from build123d import *

# Parameters (mm, degrees)
F1_DEPTH = 2.54
F2_R     = 1.27
F3_DEPTH = 25.4
F4_DEPTH = 6.35


with BuildPart() as f1:
    # F0 (on Top) → F1 (new body)
    with BuildSketch(Plane.XY):
        with BuildLine():
            Line((-17.6407694817, 88.9), (-3.0585505724, 88.9))
            ThreePointArc((-3.0585505724, 88.9), (-10.349660027, 95.0651364676), (-17.6407694817, 88.9))
        make_face()
        Polygon((-10.349660027, 0), (2.350339973, 0), (2.350339973, 56.8060912192), (-3.0585505724, 88.9), (-17.6407694817, 88.9), (-23.049660027, 56.8060912192), (-23.049660027, 0), align=None)
    extrude(amount=F1_DEPTH)

    # F2 (on face) → F3 (cut)
    with BuildSketch(Plane.XY.offset(2.54)):
        with Locations((-16.699660027, 6.35)):
            Circle(F2_R)
        with BuildLine():
            ThreePointArc((-2.729660027, 6.35), (-3.999660027, 7.62), (-5.269660027, 6.35))
            ThreePointArc((-5.269660027, 6.35), (-3.999660027, 5.08), (-2.729660027, 6.35))
        make_face()
    extrude(amount=-F3_DEPTH, mode=Mode.SUBTRACT)

    # F4 (add): a face of the model
    f4_faces = [f1.faces().sort_by_distance(p)[0] for p in [
        (-10.349660027, 0, 1.27),
    ]]
    extrude(f4_faces, amount=F4_DEPTH)


solid = f1.part
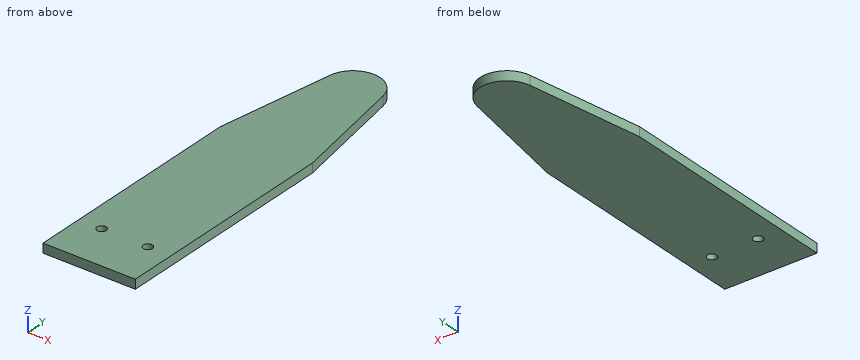
CAD build for the part. Positions are in the model's coordinates, mm. Coordinates: 2 decimals unless noted, no trailing zeros. Write each loop counter-clockwise with the first axis right and the second up, starting at its lowest first coordinate (ties: lowest second). Pieces come first, ordered by that corner, then holes. Notation, with made-up numbers: (0.5, -15) - (57.5, -15) arc R27 cw to (57.5, 1) - close; hole circle Ø1 at (59.25, 54.5). An arc over 180 degrees is marked (long way). Use a Markdown table: item, result. Add a question column.
Item 1: Flat gauge pin, fed straight in: pin 1 (1.5 mm diameter, centred on x = -16.7, y = 6.35, fed in from -Z). Where does the tip first touch, or does it go through?
Item 2: Band-saw the part on C-C, the plane x = -20.25. Give the cut face in (y, z).
Item 3: Band-saw the part on A-A, the plane y = 6.35. Give the cut face in (x, z).
Item 4: Drill centre lines: L1, parallel to Y at x = -4, z = 0.5; L2, parallel to Y at x = -17, z = 2.1; L3, parallel to Y at x = -8, z = 2.1. Where is each one in solid material? Low to high. Write a range as from..to.
Item 5: Band-saw the part on B-B, the plane z = 0.55. Give the cut face in (x, y), and give its area (3 significant figures).
Numbers:
| question | item | result |
|---|---|---|
| 1 | pin 1 | through |
| 2 | outline | (-6.35, 0) - (73.42, 0) - (73.42, 2.54) - (-6.35, 2.54) - close |
| 3 | outline | (-23.05, 0) - (-17.97, 0) - (-17.97, 2.54) - (-23.05, 2.54) - close; (-15.43, 0) - (-5.27, 0) - (-5.27, 2.54) - (-15.43, 2.54) - close; (-2.73, 0) - (2.35, 0) - (2.35, 2.54) - (-2.73, 2.54) - close |
| 4 | L1 | -6.35..5.08, 7.62..91.46 |
| 4 | L2 | -6.35..5.12, 7.58..90.9 |
| 4 | L3 | -6.35..94.68 |
| 5 | outline | (-23.05, -6.35) - (2.35, -6.35) - (2.35, 56.81) - (-3.06, 88.9) arc R7.39 ccw to (-17.64, 88.9) - (-23.05, 56.81) - close; hole circle Ø2.54 at (-16.7, 6.35); hole circle Ø2.54 at (-4, 6.35) |
| 5 | area | 2,300 mm2 |
